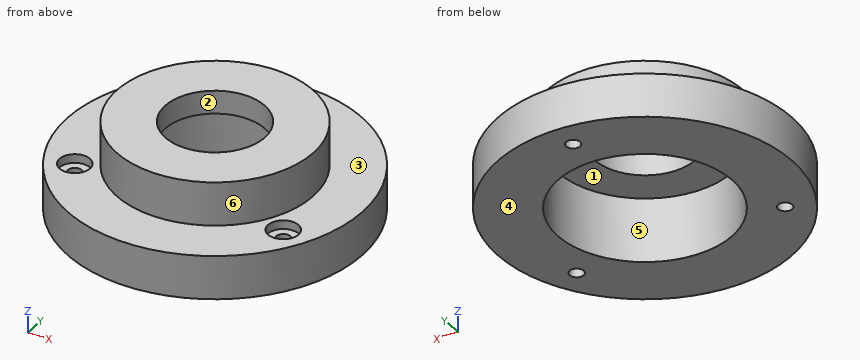
Autodesk Inventor part; units mm, degrees
ref_plane "YZ Plane" through (0, 0, 0) normal (1, 0, 0) x (0, 1, 0)
ref_plane "XZ Plane" through (0, 0, 0) normal (0, 1, 0) x (-1, 0, 0)
ref_plane "XY Plane" through (0, 0, 0) normal (0, 0, 1) x (1, 0, 0)
sketch "Sketch3" plane through (0, 0, 0) normal (0, 0, 1) x (1, 0, 0)
  circle A0 centre (0, 0) radius 33.75
  dimension "d7" = 67.5
extrude "baseExtrusion" add sketch "Sketch3" along normal blind 10
sketch "Sketch4" plane through (0, 0, 10) normal (0, 0, 1) x (1, 0, 0)
  circle A0 centre (0, 0) radius 22.5
  dimension "d10" = 45
extrude "objectiveMountExtrusion" add sketch "Sketch4" along normal blind 10
sketch "Sketch5" plane through (0, 0, 20) normal (0, 0, 1) x (1, 0, 0)
  point P0 (0, 0)
  point P1 (0, 0)
hole "objectiveThread" at (0, 0, 20) direction (0, 0, -1) diameter 22.835 end through all
sketch "Sketch6" plane through (0, 0, 0) normal (0, 0, -1) x (-1, 0, 0)
  circle A0 centre (0, 0) radius 20
  dimension "d20" = 40
extrude "objectiveClearance" cut sketch "Sketch6" against normal blind 14.7
sketch "Sketch7" plane through (0, 0, 10) normal (0, 0, 1) x (1, 0, 0)
  point P0 (0, 0)
  point P1 (0, 27.5)
  point P2 (-23.8157, -13.75)
  point P3 (23.8157, -13.75)
  dimension "d23" = 27.5
  dimension "d26" = 360
hole "holeMounts" at (0, 27.5, 10) at (-23.8157, -13.75, 10) at (23.8157, -13.75, 10) direction (0, 0, -1) diameter 3.242 end through all counterbore diameter 7 counterbore depth 2
properties part number "cylindricalObjectiveHolder"
Verification items for the finished model (mm, model axes). Face numbers are marked on the shaded views. A direction names the side the tool comes from. Coordinates: 2 decimals unless noted, no trailing zeros. Loops run counter-clockwise (first coordinate to the right, second up) from the corner with the lowest first, then second, coordinate; pieces in that order, holes last. Notation, with made-up numbers: (56, 87.5) -> (67, 87.5) arc R30 ccw to (67, 112.5) -> close; hole circle Ø1 at (31.25, 53). An arc over 180 degrees is marked (long way). Answer as CSV lines item,"result".
1) Release check for a two-part mould opening along X. For the marked faces 4, 5 and 6 record: +X half, -X half, draft (parallel to the pull), parting line (faces both ways), or undercut.
Found:
face 4,"draft"
face 5,"undercut"
face 6,"parting line"
2) Tool access check on the marked faces 1, 2 and 3. Record the directions out of +Z, -Z, +X, -X, +Y, -Y that give a thin tool (end or side, any length) a straight path to the whole face; none if there is none.
Found:
face 1,"-Z"
face 2,"+Z, -Z"
face 3,"+Z"
3) Thickness scan on L1, parallel to Y at x = 0, z = 1.5; L2, parallel to Y at x = 0, z = 9.25; L3, parallel to Y at x = 0, z = 17.95. Record the ranges inside material, lowest first. Write a range as from..to.
Found:
L1,"y = -33.75..-20, 20..25.88, 29.12..33.75"
L2,"y = -33.75..-20, 20..24, 31..33.75"
L3,"y = -22.5..-11.42, 11.42..22.5"
4) Cross-section at B-B, the plane x = 0. Record the cut outline in (y, z), then the cut area to 3 significant figures.
Found:
outline,"(-33.75, 0) -> (-20, 0) -> (-20, 14.7) -> (-11.42, 14.7) -> (-11.42, 20) -> (-22.5, 20) -> (-22.5, 10) -> (-33.75, 10) -> close; (11.42, 14.7) -> (20, 14.7) -> (20, 0) -> (25.88, 0) -> (25.88, 8) -> (24, 8) -> (24, 10) -> (22.5, 10) -> (22.5, 20) -> (11.42, 20) -> close; (29.12, 0) -> (33.75, 0) -> (33.75, 10) -> (31, 10) -> (31, 8) -> (29.12, 8) -> close"
area,"376 mm2"
5) Cross-section at C-C, the plane z = 18. Record the cut outline in (x, y) (1 decimal).
Found:
outline,"circle Ø45 at (0, 0); hole circle Ø22.8 at (0, 0)"
6) Cross-section at A-A, the plane y = 0. Record the cut outline in (x, z).
Found:
outline,"(-33.75, 0) -> (-20, 0) -> (-20, 14.7) -> (-11.42, 14.7) -> (-11.42, 20) -> (-22.5, 20) -> (-22.5, 10) -> (-33.75, 10) -> close; (11.42, 14.7) -> (20, 14.7) -> (20, 0) -> (33.75, 0) -> (33.75, 10) -> (22.5, 10) -> (22.5, 20) -> (11.42, 20) -> close"
7) Cross-section at D-D, the plane y = -13.75. Record the cut outline in (x, z), then the cut area to 3 significant figures.
Found:
outline,"(-30.82, 0) -> (-25.44, 0) -> (-25.44, 8) -> (-27.32, 8) -> (-27.32, 10) -> (-30.82, 10) -> close; (-22.19, 0) -> (-14.52, 0) -> (-14.52, 14.7) -> (14.52, 14.7) -> (14.52, 0) -> (22.19, 0) -> (22.19, 8) -> (20.32, 8) -> (20.32, 10) -> (17.81, 10) -> (17.81, 20) -> (-17.81, 20) -> (-17.81, 10) -> (-20.32, 10) -> (-20.32, 8) -> (-22.19, 8) -> close; (25.44, 0) -> (30.82, 0) -> (30.82, 10) -> (27.32, 10) -> (27.32, 8) -> (25.44, 8) -> close"
area,"466 mm2"
8) Depth check by flat-ended pin: pin 1 (6.5 mm diameter, centred on x = 0, y = 27.5, fed in from +Z); pin 2 (7.5 mm diameter, centred on x = -1.5, y = 26.5, fed in from +Z); pin 3 (2 mm diameter, centred on y = 5, z = 14.5, fed in from -X); pin 4 (20.5 mm diameter, centred on x = 0, y = 0, fed in from -Z). Enter the tip coordinate at first touch or a pass-through.
Found:
pin 1,"stops at z = 8"
pin 2,"stops at z = 10"
pin 3,"stops at x = -22.14"
pin 4,"passes through"
